CAD build for the part. Positions are in the model's coordinates, mm. Face numbers are marked on the shaded views. A direction names the side the tool comes from. Coordinates: 2 decimals unless noted, no trailing zeros. Write each loop counter-clockwise with the first axis right and the second up, starting at its lowest first coordinate (ties: lowest second). Pieces come first, ordered by that corner, then holes. Notation, with made-up numbers: M 79,28 L 114,28 A23 cw 114,65 Z; hole C -34,57 d5. An arc over 180 degrees is marked long. Put each result on its own line as item: value. Start each with the question number.
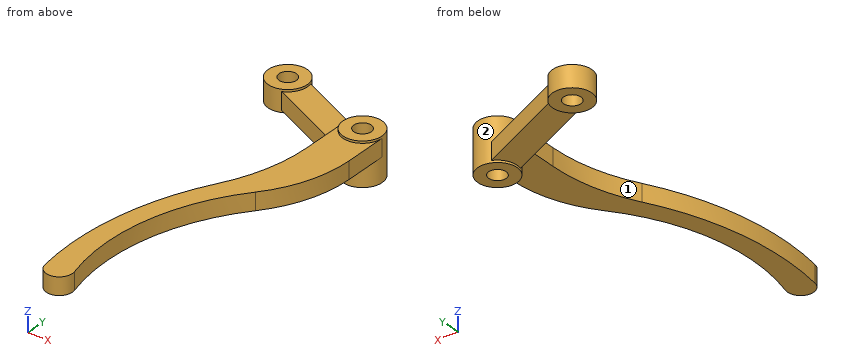
```python
from build123d import *

# Parameters (mm, degrees)
SKETCH_1_R        = 9
SKETCH_1_R_2      = 4
EXTRUDE_1_DEPTH   = 10
EXTRUDE_1_2_DEPTH = 10
EXTRUDE_START     = -9
EXTRUDE_2_DEPTH   = 8
EXTRUDE_START_2   = 1
EXTRUDE_3_DEPTH   = 8
SKETCH_5_R        = 9
SKETCH_5_R_2      = 4
EXTRUDE_4_DEPTH   = 10


with BuildPart() as part:
    # Sketch 1 → Extrude 1 (new body)
    with BuildSketch(Plane.XY):
        Circle(SKETCH_1_R)
        Circle(SKETCH_1_R_2, mode=Mode.SUBTRACT)
    extrude(amount=EXTRUDE_1_DEPTH)



with BuildPart() as body_2:
    # Sketch 1 → Extrude 1 2 (new body)
    with BuildSketch(Plane.XY):
        with Locations((-54.075649928, 25.996616797)):
            Circle(SKETCH_1_R)
        with Locations((-54.075649928, 25.996616797)):
            Circle(SKETCH_1_R_2, mode=Mode.SUBTRACT)
    extrude(amount=EXTRUDE_1_2_DEPTH)


with BuildPart() as part_1:
    add(part.part)

    add(body_2.part)  # Extrude 2 merges body 2
    # Sketch 2 → Extrude 2 (add)
    with BuildSketch(Plane.XY.offset(10).offset(EXTRUDE_START)):
        with BuildLine():
            Line((-50.629470149, 17.682541688), (-8.645503138, -2.501054876))
            ThreePointArc((-8.645503138, -2.501054876), (-8.111347489, 3.89949252), (-3.446179779, 8.31407511))
            Line((-3.446179779, 8.31407511), (-45.43014679, 28.497671673))
            ThreePointArc((-45.43014679, 28.497671673), (-45.964302438, 22.097124278), (-50.629470149, 17.682541688))
        make_face()
    extrude(amount=EXTRUDE_2_DEPTH)



with BuildPart() as body_2_2:
    # Sketch 4 → Extrude 3 (new body)
    with BuildSketch(Plane.XY.offset(10).offset(EXTRUDE_START_2)):
        with BuildLine():
            Line((-9, 0), (-9, -22))
            ThreePointArc((-9, -22), (-11.716267411, -42.669414049), (-19.680616928, -61.935236704))
            ThreePointArc((-19.680616928, -61.935236704), (-34.813823432, -102.892867464), (-35.532086941, -146.550920033))
            ThreePointArc((-35.532086941, -146.550920033), (-28.368122981, -151.512581419), (-23.805971944, -144.087809285))
            ThreePointArc((-23.805971944, -144.087809285), (-24.813823432, -99.040827427), (-4.952136173, -58.596300996))
            ThreePointArc((-4.952136173, -58.596300996), (5.404218945, -40.589645691), (9, -20.130806888))
            Line((9, -20.130806888), (9, 0))
            ThreePointArc((9, 0), (0, -9), (-9, 0))
        make_face()
    extrude(amount=EXTRUDE_3_DEPTH)


with BuildPart() as part_2:
    add(part_1.part)

    add(body_2_2.part)  # Extrude 4 merges body 2 2
    # Sketch 5 → Extrude 4 (add)
    with BuildSketch(Plane.XY.offset(10)):
        Circle(SKETCH_5_R)
        Circle(SKETCH_5_R_2, mode=Mode.SUBTRACT)
    extrude(amount=EXTRUDE_4_DEPTH)


solid = part_2.part
```
(1) Slice it at B-B, the plane z = 16. Write the cut outline in (x, y), then the cut area to 3 significant figures.
(2) Slice it at D-D, the plane x = -13.5. Write the cut outline in (y, z), then the cut area to 3 significant figures.
(3) Slice it at A-A, the plane x = 0. Write the cut outline in (y, z).
(4) Slice it at C-C, the plane y = -99. Write the cut outline in (x, z).
(5) Which spindle directions (+Z, -Z, +X, -X, +Y, -Y) get a long thin tool onto all of the face, cutting with end or side? Do the marked faces 1 and 2. Say none if no direction does.
(6) Drill centre lines: line 1 (Y direction, x = 0, z = 9); line 2 (X direction, y = 3, z = 9.25); line 3 (Y direction, x = 0, z = 12). Where is each one in solid material? Low to high. Write a range as [from, to].
(7) Drop flat-ended pins along their axis: pin 1 (9 mm diameter, centred on x = -58, y = 29.5, fed in from +Z); pin 2 (9.5 mm diameter, centred on x = -24, y = 5.5, fed in from -Z); pin 3 (4 mm diameter, centred on y = -10, z = 15.5, fed in from -X). Give the stop position or say it passes through.
Result set:
1. outline: M -35.53,-146.55 A6 ccw long -23.81,-144.09 A95 cw -4.95,-58.6 A60 ccw 9,-20.13 L 9,0 A9 ccw -9,0 L -9,-22 A80 cw -19.68,-61.94 A130 ccw Z; hole C 0,0 d8
1. area: 2,020 mm^2
2. outline: M -70.61,11 L -48.45,11 L -48.45,19 L -70.61,19 Z; M -0.17,1 L 13.15,1 L 13.15,9 L -0.17,9 Z
2. area: 284 mm^2
3. outline: M -51.74,11 L -9,11 L -9,0 L -4,0 L -4,20 L -9,20 L -9,19 L -51.74,19 Z; M 4,0 L 9,0 L 9,20 L 4,20 Z
4. outline: M -34.02,11 L -24.8,11 L -24.8,19 L -34.02,19 Z
5. face 1: +Z, -Z, -X, +Y
5. face 2: none
6. line 1: y = [-9, -4], [4, 9]
6. line 2: x = [-8.49, -2.65], [2.65, 8.49]
6. line 3: y = [-51.74, -4], [4, 9]
7. pin 1: stops at z = 10
7. pin 2: stops at z = 1
7. pin 3: stops at x = -9
